from build123d import *

# Parameters (mm, degrees)
F0_R          = 0.9
F1_DEPTH      = 18.725
F1_DEPTH_BACK = 18.725
F2_W          = 27.45
F2_H          = 10
F3_DEPTH      = 25
F3_DEPTH_BACK = 25
F4_DEPTH      = 5
F4_DEPTH_BACK = 5


with BuildPart() as f1:
    # F0 (on Right) → F1 (new body, two sides)
    with BuildSketch(Plane.YZ) as f1_sk:
        with BuildLine():
            Line((-35, 2.5), (-28, 2.5))
            Line((-28, 2.5), (-28, 9.1788107529))
            ThreePointArc((-28, 9.1788107529), (-31.5, 12.6788107529), (-35, 9.1788107529))
            Line((-35, 9.1788107529), (-35, 2.5))
        make_face()
        with Locations((-31.5, 7.5)):
            Circle(F0_R, mode=Mode.SUBTRACT)
        Polygon((35.0000000196, 7.8434e-06), (35.0000000196, 2.5), (-28, 2.5), (-35, 2.5), (-35.0062623424, 7.8434e-06), align=None)
    extrude(amount=F1_DEPTH)
    extrude(f1_sk.sketch, amount=-F1_DEPTH_BACK)

    # F2 (on Top) → F3 (cut, two sides)
    with BuildSketch(Plane.XY) as f3_sk:
        with Locations((0, -33)):
            Rectangle(F2_W, F2_H)
    extrude(amount=F3_DEPTH, mode=Mode.SUBTRACT)
    extrude(f3_sk.sketch, amount=-F3_DEPTH_BACK, mode=Mode.SUBTRACT)

    # F2 (on Top) → F4 (cut, two sides)
    with BuildSketch(Plane.XY) as f4_sk:
        Polygon((15, 17), (15, 10), (25, 10), (25, 31), (15, 31), (15, 24), align=None)
        Polygon((-25, 10), (-15, 10), (-15, 17), (-15, 24), (-15, 31), (-25, 31), align=None)
        Polygon((-15, 17), (-15, 10), (-8, 10), align=None)
        Polygon((-15, 31), (-15, 24), (-8, 31), align=None)
        Polygon((8, 10), (15, 10), (15, 17), align=None)
        Polygon((8, 31), (15, 24), (15, 31), align=None)
        Polygon((15, 31), (25, 31), (25, 38), (1, 38), (8, 31), align=None)
        Polygon((25, 10), (15, 10), (8, 10), (25, -7), align=None)
        Polygon((-8, 10), (-15, 10), (-25, 10), (-25, -7), align=None)
        Polygon((-25, 38), (-25, 31), (-15, 31), (-8, 31), (-1, 38), align=None)
    extrude(amount=-F4_DEPTH, mode=Mode.SUBTRACT)
    extrude(f4_sk.sketch, amount=F4_DEPTH_BACK, mode=Mode.SUBTRACT)


solid = f1.part
The model under review builds one solid part; all positions refer to its coordinate system, in mm. A direction names the side the tool comes from. Give positions to 0.01 mm unless a question says otherwise; leave off trailing zeros. Loops run counter-clockwise (first coordinate to the right, second up) from the corner with the lowest first, then second, coordinate; pieces in that order, holes last. Notation, with made-up numbers: (17, 34.25) -> (39, 34.25) arc R26 cw to (39, 59.25) -> close; hole circle Ø1 at (59, 46). An arc over 180 degrees is marked (long way). Write each question's results on one line, items separated by ' | '.
1) For line 1 along Y through (x, z) = (17.3, 7.5); line 2 along X through (y, z) = (-30, 10.75) (3 decimals); line 3 along Z through (x, y) = (-15.7, -31.5), list the stretches that pass through material, from the lowest coordinate up. Write a range as from..to.
Conclusion:
line 1: y = -35..-32.4, -30.6..-28 | line 2: x = -18.725..-13.725, 13.725..18.725 | line 3: z = 0..6.6, 8.4..12.68
2) Draft analysis for pull direction X (two halves, no side actions). For faces 1 (the face through (-18.725, -26, 2)), 2 (the face through (-13.725, -32, 6)), 3 (the face through (-16, -35, 6)), state which applies: pulls with the +X half, pulls with the -X half, needs draft (parallel to the pull), parting line crosses it, or undercut.
Conclusion:
face 1: pulls with the -X half | face 2: undercut | face 3: needs draft
3) Take a section at C-C, the plane x = 2. Give the boundary of the cut face in (y, z).
Conclusion:
outline: (-28, 0) -> (35, 0) -> (35, 2.5) -> (-28, 2.5) -> close
4) Tool access review of faces 4 (the face through (13.725, -32, 6)), 5 (the face through (-13, 5, 1)), 6 (the face through (13, 5, 1)): name each direction out of +Z, -Z, +X, -X, +Y, -Y from which nothing blocks a thin tool from reaching the whole face with its end or side.
Conclusion:
face 4: +Z, -Z, -Y | face 5: +Z, -Z, -X | face 6: +Z, -Z, +X
5) Take a section at D-D, the plane y = 28.5. Give the boundary of the cut face in (x, z), plus the area to 3 significant figures.
Conclusion:
outline: (-10.5, 0) -> (10.5, 0) -> (10.5, 2.5) -> (-10.5, 2.5) -> close | area: 52.5 mm^2
6) Take a section at B-B, the plane y = -31.5. Give the boundary of the cut face in (x, z) (3 decimals).
Conclusion:
outline: (-18.725, 0) -> (-13.725, 0) -> (-13.725, 6.6) -> (-18.725, 6.6) -> close; (-18.725, 8.4) -> (-13.725, 8.4) -> (-13.725, 12.679) -> (-18.725, 12.679) -> close; (13.725, 0) -> (18.725, 0) -> (18.725, 6.6) -> (13.725, 6.6) -> close; (13.725, 8.4) -> (18.725, 8.4) -> (18.725, 12.679) -> (13.725, 12.679) -> close
7) Take a section at A-A, the plane z = 4.5. Give the boundary of the cut face in (x, y) (3 decimals).
Conclusion:
outline: (-18.725, -35) -> (-13.725, -35) -> (-13.725, -28) -> (-18.725, -28) -> close; (13.725, -35) -> (18.725, -35) -> (18.725, -28) -> (13.725, -28) -> close
8) Insertion check: pin 1 Ø1.5 at (y, z) = (-19, 3) entering from -X (3 decimals); pin 2 Ø6 at (x, y) = (-10.5, 5) entering from +Z; pin 3 Ø5 at (x, z) = (10, 10) entering from +Y; pin 4 Ø2 at (y, z) = (21.5, 1.5) entering from -X. Each pin has a flat end and moves straight along its axis. Give the tip position at first contact, or say it passes through.
Conclusion:
pin 1: stops at x = -18.725 | pin 2: stops at z = 2.5 | pin 3: passes through | pin 4: stops at x = -15
